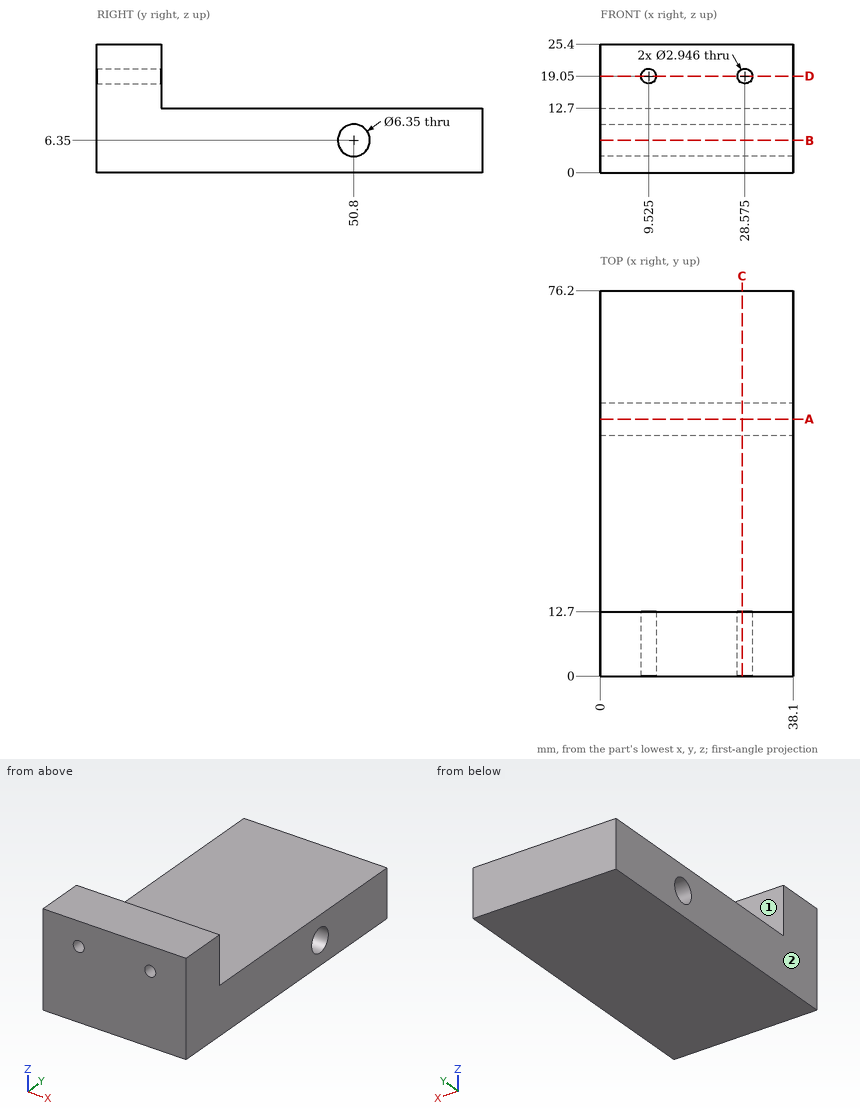
Geometry check sheet. Reference: drawing and pictorial views, mm from the part's lowest x, y, z. A direction names the side the tool comes from. Coordinates: 2 decimals unless noted, no trailing zeros. Write each loop counter-clockwise with the first axis right and the second up, starting at its lowest first coordinate (ties: lowest second). Pieces come first, ordered by that corner, then holes. Notation, with made-up numbers: M -16.5,55 L 10.5,55 A21 ccw 10.5,60 Z; hole C 45.25,81 d5. An arc over 180 degrees is marked long. Write item = value, one per line. Start each with the question number.
1. Sectioned sample at C-C (x = 28). State how many separate pieces and enclosed holes the cut face has, then the cut area to 3 significant figures.
2. Go/stop test with flat-tipped pins: pin 1 (12 mm diameter, centred on x = 21, y = 29, fed in from +Z); pin 2 (8 mm diameter, centred on y = 12.5, z = 5.5, fed in from -X); pin 3 (4 mm diameter, centred on x = 11.5, z = 18, fed in from +Y). Record where each tip stops, or that it passes through.
3. Sectioned sample at D-D (z = 19.05). Record the cut outline in (x, y), then the cut area to 3 significant figures.
4. Sectioned sample at A-A (y = 50.8). Record the cut outline in (x, z) (1 decimal), then the cut area to 3 significant figures.
5. Sectioned sample at B-B (z = 6.35). Record the cut outline in (x, y) (1 decimal).
6. Tool access check on the marked faces 1 and 2. Record the directions out of +Z, -Z, +X, -X, +Y, -Y that give a thin tool (end or side, any length) a straight path to the whole face; none if there is none.
7. Thickness scan on probe 1 along X at (y, z) = (9.5, 19.05); probe 2 along Z at (x, y) = (22.5, 51); probe 3 along Y at (x, z) = (11.5, 6.35) (1 decimal). Record the ranges inside material, lowest first.
The answers:
q1.separate_pieces = 2
q1.enclosed_holes = 1
q1.area = 1,060 mm²
q2.pin_1 = 12.7
q2.pin_2 = 0
q2.pin_3 = 12.7
q3.outline = M 0,0 L 8.05,0 L 8.05,12.7 L 0,12.7 Z; M 11,0 L 27.1,0 L 27.1,12.7 L 11,12.7 Z; M 30.05,0 L 38.1,0 L 38.1,12.7 L 30.05,12.7 Z
q3.area = 409 mm²
q4.outline = M 0,0 L 38.1,0 L 38.1,3.2 L 0,3.2 Z; M 0,9.5 L 38.1,9.5 L 38.1,12.7 L 0,12.7 Z
q4.area = 242 mm²
q5.outline = M 0,0 L 38.1,0 L 38.1,47.6 L 0,47.6 Z; M 0,54 L 38.1,54 L 38.1,76.2 L 0,76.2 Z
q6.face_1 = +Z, +X, -X, +Y
q6.face_2 = +Z, -Z, -X, +Y, -Y
q7.probe_1 = 0 to 8.05, 11 to 27.1, 30.05 to 38.1
q7.probe_2 = 0 to 3.18, 9.52 to 12.7
q7.probe_3 = 0 to 47.6, 54 to 76.2
